from build123d import *

# Parameters (mm, degrees)
SKETCH1_R                   = 15.875
BOSS_EXTRUDE1_DEPTH         = 12.7
SKETCH2_R                   = 0.7493
CUT_EXTRUDE1_DEPTH          = 20
SKETCH3_R                   = 1.2192
CUT_EXTRUDE3_DEPTH          = 26.793821935
CUT_EXTRUDE4_START          = -20
CUT_EXTRUDE4_DEPTH          = 20
CIRPATTERN1_COUNT           = 6
F_32_0_116_DIAMETER_HOLE2_D = 2.9464


with BuildPart() as part:
    # Sketch1 → Boss-Extrude1 (new body)
    with BuildSketch(Plane(origin=(0, 0, 0), x_dir=(1, 0, 0), z_dir=(0, 1, 0))):
        with Locations(Location((0, 0, 0), (0, 0, 270))):
            Circle(SKETCH1_R)
    extrude(amount=BOSS_EXTRUDE1_DEPTH)

    # Sketch2 → Cut-Extrude1 (cut)
    with BuildSketch(Plane(origin=(0, 12.7, 0), x_dir=(1, 0, 0), z_dir=(0, 1, 0))):
        with Locations(Location((0, 0, 0), (0, 0, 270))):
            Circle(SKETCH2_R)
    extrude(amount=-CUT_EXTRUDE1_DEPTH, mode=Mode.SUBTRACT)

    # Sketch3 → Cut-Extrude3 (cut, through all)
    with BuildSketch(Plane(origin=(0, 12.7, 0), x_dir=(1, 0, 0), z_dir=(0, 1, 0))):
        with Locations(Location((0, 12.7, 0), (0, 0, 270))):
            Circle(SKETCH3_R)
    cut_extrude3 = extrude(amount=-CUT_EXTRUDE3_DEPTH, mode=Mode.SUBTRACT)

    # Sketch4 → Cut-Extrude4 (cut)
    with BuildSketch(Plane(origin=(0, 12.7, 0), x_dir=(1, 0, 0), z_dir=(0, 1, 0)).offset(CUT_EXTRUDE4_START)):
        with BuildLine():
            ThreePointArc((12.7, 3.175), (9.525, 0), (12.7, -3.175))
            Line((12.7, -3.175), (12.7, 3.175))
        make_face()
        with BuildLine():
            Line((12.7, 3.175), (12.7, -3.175))
            ThreePointArc((12.7, -3.175), (14.94506403, -2.24506403), (15.875, 0))
            ThreePointArc((15.875, 0), (14.94506403, 2.24506403), (12.7, 3.175))
        make_face()
        with BuildLine():
            ThreePointArc((15.875, 0), (15.794611429, -1.595579772), (15.554259867, -3.175))
            Line((15.554259867, -3.175), (20.958617126, -3.175))
            Line((20.958617126, -3.175), (20.958617126, 3.175))
            Line((20.958617126, 3.175), (15.554259867, 3.175))
            ThreePointArc((15.554259867, 3.175), (15.794611429, 1.595579772), (15.875, 0))
        make_face()
        with BuildLine():
            Line((15.554259867, 3.175), (12.7, 3.175))
            ThreePointArc((12.7, 3.175), (14.94506403, 2.24506403), (15.875, 0))
            ThreePointArc((15.875, 0), (15.794611429, 1.595579772), (15.554259867, 3.175))
        make_face()
        with BuildLine():
            ThreePointArc((15.875, 0), (14.94506403, -2.24506403), (12.7, -3.175))
            Line((12.7, -3.175), (15.554259867, -3.175))
            ThreePointArc((15.554259867, -3.175), (15.794611429, -1.595579772), (15.875, 0))
        make_face()
    cut_extrude4 = extrude(amount=CUT_EXTRUDE4_DEPTH, mode=Mode.SUBTRACT)

    # CirPattern1: Cut-Extrude3, Cut-Extrude4 ×6 about axis
    cirpattern1_axis = Axis((0, 0, 0), (0, 1, 0))
    add([cut_extrude3.rotate(cirpattern1_axis, i * 360 / CIRPATTERN1_COUNT) for i in range(1, CIRPATTERN1_COUNT)], mode=Mode.SUBTRACT)
    add([cut_extrude4.rotate(cirpattern1_axis, i * 360 / CIRPATTERN1_COUNT) for i in range(1, CIRPATTERN1_COUNT)], mode=Mode.SUBTRACT)

    # #32 (0.116) Diameter Hole2 (through all)
    with Locations(Plane(origin=(0, 0, 0), x_dir=(-1, 0, 0), z_dir=(0, -1, 0))):
        with Locations((5.291415217, -3.055), (-5.291415217, 3.055)):
            Hole(F_32_0_116_DIAMETER_HOLE2_D / 2)


solid = part.part
Geometry check sheet. Reference: the model listing, model coordinates, mm. A direction names the side the tool comes from. Coordinates: 2 decimals unless noted, no trailing zeros. Order: outer loops, then holes, each group sorted by start corner. A loop starts at its lowest first (then second) coordinate and runs counter-clockwise, first axis right, second up. Notation, with made-up numbers: (46, 42.25) - (53, 42.25) arc R21 ccw to (53, 76.25) - close; hole circle Ø8 at (81.25, 79). An arc over 180 degrees is marked (long way). One line per item, written item: value.
(1) Access from +Z, -Z, +X, -X, +Y, -Y to the whole of each face (thin tool, end or side, straight path). Record for faces 1 (the face through (9.803, 6.261, -10.63)), 2 (the face through (-4.823, 6.261, -8.215)), 3 (the face through (-14, 6, -3.175)), 4 (the face through (-9.803, 6.261, 10.63)), 5 (the face through (4.3, 6.3, 13.8)).
Data:
face 1: -Z, +Y, -Y
face 2: +Y, -Y
face 3: -X, +Y, -Y
face 4: +Z, +Y, -Y
face 5: +X, +Y, -Y
(2) Release check for a two-part mould opening along X. For faces 6 (the face through (-9.526, 6.261, 0.07)), 7 (the face through (-4.702, 6.261, 8.284)), 8 (the face through (0.072, 6.261, -15.875)) record: +X half, -X half, draft (parallel to the pull), parting line (faces both ways), or undercut.
Data:
face 6: -X half
face 7: undercut
face 8: parting line
(3) Sectioned sample at D-D (y = 8.25). Count the separate pieces of the cut face and the enclosed holes in it, and give its area (3 significant figures).
Data:
separate pieces: 1
enclosed holes: 9
area: 536 mm^2
(4) Thickness scan on probe 1 along X at (y, z) = (5.75, 6.35); probe 2 along X at (y, z) = (11, 9.5); probe 3 along X at (y, z) = (5.75, 0) (3 decimals). Record the ranges inside material, lowest first. Write a range as from..to.
Data:
probe 1: x = -14.55..-12.22, -9.78..9.78, 12.22..14.55
probe 2: x = -12.72..-9.15, -3.55..3.55, 9.15..12.72
probe 3: x = -9.525..-0.749, 0.749..9.525
(5) Sectioned sample at B-B (z = 0). Enter the section's corners in (x, y) (3 decimals), and give its area (3 significant figures).
Data:
outline: (-9.525, 0) - (-0.749, 0) - (-0.749, 12.7) - (-9.525, 12.7) - close; (0.749, 0) - (9.525, 0) - (9.525, 12.7) - (0.749, 12.7) - close
area: 223 mm^2
(6) Sectioned sample at A-A (x = 0). Enter the section's corners in (y, z) (3 decimals), and give its area (3 significant figures).
Data:
outline: (0, -15.875) - (12.7, -15.875) - (12.7, -13.919) - (0, -13.919) - close; (0, -11.481) - (12.7, -11.481) - (12.7, -0.749) - (0, -0.749) - close; (0, 0.749) - (12.7, 0.749) - (12.7, 11.481) - (0, 11.481) - close; (0, 13.919) - (12.7, 13.919) - (12.7, 15.875) - (0, 15.875) - close
area: 322 mm^2
(7) Depth check by flat-ended pin: pin 1 Ø3 at (y, z) = (6, -1) entering from +X; pin 2 Ø2.5 at (x, z) = (5.29, -3.06) entering from +Y; pin 3 Ø1.4 at (x, y) = (-14.5, 9.5) entering from -Z; pin 4 Ø0.9 at (x, y) = (-13.5, 7.5) entering from +Z. Enter the tip coordinate at first touch or a pass-through.
Data:
pin 1: stops at x = 10.74
pin 2: passes through
pin 3: stops at z = -7.85
pin 4: stops at z = 9.04
(8) Sectioned sample at C-C (x = 5.5). Enter the section's corners in (y, z).
Data:
outline: (0, -7.94) - (12.7, -7.94) - (12.7, -4.51) - (0, -4.51) - close; (0, -1.6) - (12.7, -1.6) - (12.7, 7.94) - (0, 7.94) - close
